Geometry: final body of the model. Coordinates: model frame, mm. A direction names the side the tool comes from. Give positions to 0.01 mm unless a question says otherwise; leave off trailing zeros. Write each loop counter-clockwise with the first axis right and the second up, starting at its lowest first coordinate (ties: lowest second). Pieces come first, ordered by that corner, then holes.
```python
from build123d import *

# Parameters (mm, degrees)
BOSS_EXTRUDE1_DEPTH = 1.6
FILLET1_R           = 2.5
SKETCH15_R          = 2.5
CUT_EXTRUDE5_DEPTH  = 2.6
SKETCH16_R          = 0.3
CUT_EXTRUDE6_DEPTH  = 2.6


with BuildPart() as part:
    # Sketch1 → Boss-Extrude1 (new body)
    with BuildSketch(Plane(origin=(0, 0, 0), x_dir=(1, 0, 0), z_dir=(0, 1, 0))):
        Polygon((-49, 6.540916192), (-42.459083808, 0), (42.459083808, 0), (49, 6.540916192), (49, 50.753104052), (49, 52.874424396), (46.028679707, 55.845744689), (46.028679707, 57.999655213), (49, 60.970975506), (49, 63.09229585), (49, 107.30448371), (42.459083808, 113.845399902), (42.459083808, 121.922399609), (-42.459083808, 121.922399609), (-42.459083808, 113.845399902), (-49, 107.30448371), (-49, 63.09229585), (-44.528679707, 58.620975557), (-44.528679707, 55.224424345), (-49, 50.753104052), align=None)
    extrude(amount=BOSS_EXTRUDE1_DEPTH)

    # Fillet1
    fillet1_edges = [part.edges().sort_by_distance(p)[0] for p in [
        (49, 0.8, -6.540916192),
        (42.459083808, 0.8, 0),
        (-42.459083808, 0.8, 0),
        (-49, 0.8, -6.540916192),
        (-49, 0.8, -50.753104052),
        (-44.528679707, 0.8, -55.224424345),
        (-44.528679707, 0.8, -58.620975557),
        (-49, 0.8, -63.09229585),
        (-49, 0.8, -107.30448371),
        (-42.459083808, 0.8, -113.845399902),
        (42.459083808, 0.8, -113.845399902),
        (49, 0.8, -107.30448371),
        (49, 0.8, -60.970975506),
        (46.028679707, 0.8, -57.999655213),
        (46.028679707, 0.8, -55.845744689),
        (49, 0.8, -52.874424396),
    ]]
    fillet(fillet1_edges, radius=FILLET1_R)

    # Sketch15 → Cut-Extrude5 (cut, through all)
    with BuildSketch(Plane(origin=(0, 1.6, 0), x_dir=(1, 0, 0), z_dir=(0, 1, 0))):
        with Locations((-37.846, 9.4767)):
            Circle(SKETCH15_R)
    extrude(amount=-CUT_EXTRUDE5_DEPTH, mode=Mode.SUBTRACT)

    # Sketch16 → Cut-Extrude6 (cut, through all)
    with BuildSketch(Plane(origin=(0, 1.6, 0), x_dir=(1, 0, 0), z_dir=(0, 1, 0))):
        with Locations((-29.13, 119.672399609)):
            Circle(SKETCH16_R)
        with Locations((-27.86, 119.672399609)):
            Circle(SKETCH16_R)
        with Locations((-26.59, 119.672399609)):
            Circle(SKETCH16_R)
        with Locations((-25.32, 119.672399609)):
            Circle(SKETCH16_R)
        with Locations((-24.05, 119.672399609)):
            Circle(SKETCH16_R)
        with Locations((-22.78, 119.672399609)):
            Circle(SKETCH16_R)
        with Locations((-21.51, 119.672399609)):
            Circle(SKETCH16_R)
        with Locations((-20.24, 119.672399609)):
            Circle(SKETCH16_R)
        with Locations((-18.97, 119.672399609)):
            Circle(SKETCH16_R)
        with Locations((-17.7, 119.672399609)):
            Circle(SKETCH16_R)
        with Locations((-16.43, 119.672399609)):
            Circle(SKETCH16_R)
        with Locations((-15.16, 119.672399609)):
            Circle(SKETCH16_R)
        with Locations((-13.89, 119.672399609)):
            Circle(SKETCH16_R)
        with Locations((-12.62, 119.672399609)):
            Circle(SKETCH16_R)
        with Locations((-11.35, 119.672399609)):
            Circle(SKETCH16_R)
        with Locations((-10.08, 119.672399609)):
            Circle(SKETCH16_R)
        with Locations((-8.81, 119.672399609)):
            Circle(SKETCH16_R)
        with Locations((-7.54, 119.672399609)):
            Circle(SKETCH16_R)
        with Locations((-6.27, 119.672399609)):
            Circle(SKETCH16_R)
        with Locations((-5, 119.672399609)):
            Circle(SKETCH16_R)
        with Locations((5, 119.672399609)):
            Circle(SKETCH16_R)
        with Locations((6.27, 119.672399609)):
            Circle(SKETCH16_R)
        with Locations((7.54, 119.672399609)):
            Circle(SKETCH16_R)
        with Locations((8.81, 119.672399609)):
            Circle(SKETCH16_R)
        with Locations((10.08, 119.672399609)):
            Circle(SKETCH16_R)
        with Locations((11.35, 119.672399609)):
            Circle(SKETCH16_R)
        with Locations((12.62, 119.672399609)):
            Circle(SKETCH16_R)
        with Locations((13.89, 119.672399609)):
            Circle(SKETCH16_R)
        with Locations((15.16, 119.672399609)):
            Circle(SKETCH16_R)
        with Locations((16.43, 119.672399609)):
            Circle(SKETCH16_R)
        with Locations((17.7, 119.672399609)):
            Circle(SKETCH16_R)
        with Locations((18.97, 119.672399609)):
            Circle(SKETCH16_R)
        with Locations((20.24, 119.672399609)):
            Circle(SKETCH16_R)
        with Locations((21.51, 119.672399609)):
            Circle(SKETCH16_R)
        with Locations((22.78, 119.672399609)):
            Circle(SKETCH16_R)
        with Locations((24.05, 119.672399609)):
            Circle(SKETCH16_R)
        with Locations((25.32, 119.672399609)):
            Circle(SKETCH16_R)
        with Locations((26.59, 119.672399609)):
            Circle(SKETCH16_R)
        with Locations((27.86, 119.672399609)):
            Circle(SKETCH16_R)
        with Locations((29.13, 119.672399609)):
            Circle(SKETCH16_R)
    extrude(amount=-CUT_EXTRUDE6_DEPTH, mode=Mode.SUBTRACT)


solid = part.part
```
Item 1: Pin query (flat end, axial travel): pin 1 Ø0.5 at (y, z) = (1, -118.5) entering from +X. Return the tip coordinate at first contact, or that it passes through.
Found:
pin 1: stops at x = 42.46
Item 2: Section A-A, the plane x = -39. Return the cut outline in (y, z).
Found:
outline: (0, -121.92) - (1.6, -121.92) - (1.6, -11.69) - (0, -11.69) - close; (0, -7.26) - (1.6, -7.26) - (1.6, 0) - (0, 0) - close
Item 3: Reachability of faces 4 (the face through (-46.743, 0.789, -53.01)), 5 (the face through (-1, 1.6, -62)) from +Z, -Z, +X, -X, +Y, -Y: full face, straight path, thin tool, end or side. Return the list, or none.
Found:
face 4: -X, +Y, -Y
face 5: +Z, -Z, +X, -X, +Y
Item 4: Line query: L1, parallel to Z at x = -24.05, y = 0.6; L2, parallel to Z at x = -29, y = 1.35; L3, parallel to X at y = 0.1, z = -10.5. Output: solid intervals per line, ascending.
Found:
L1: z = -121.92 to -119.97, -119.37 to 0
L2: z = -121.92 to -119.94, -119.4 to 0
L3: x = -49 to -40.13, -35.57 to 49
Item 5: Pull-direction query (Z, two-part tool) for faces 1 (the face through (-1, 0, -62)), 2 (the face through (-35.461, 0.811, -10.228)), 3 (the face through (-45.694, 0.789, -110.61)); classes: +Z half, -Z half, draft (parallel to the pull), parting line (faces both ways), or undercut.
Found:
face 1: draft
face 2: undercut
face 3: -Z half
Item 6: Section B-B, the plane y = 0.4. State how many separate pieces and enclosed holes the cut face has, plus the area to 3 significant figures.
Found:
separate pieces: 1
enclosed holes: 41
area: 11,700 mm2
